```python
from build123d import *

# Parameters (mm, degrees)
BOSS_EXTRUDE1_DEPTH = 2
CUT_EXTRUDE1_REACH  = 43.449
SKETCH2_R           = 1
SKETCH3_W           = 42.8
SKETCH3_H           = 53.28
CUT_EXTRUDE2_DEPTH  = 1
SKETCH4_W           = 1.5
SKETCH4_H           = 57.28
BOSS_EXTRUDE2_DEPTH = 3.5
SKETCH5_W           = 1
SKETCH5_H           = 3
CUT_EXTRUDE3_DEPTH  = 16.633
CHAMFER1_SIZE       = 1
CHAMFER2_SIZE       = 2.5
CHAMFER3_SIZE       = 1.5
CHAMFER4_SIZE       = 1.5


# Some blends are built 0.0001 mm under size
with BuildPart() as part:
    # Sketch1 → Boss-Extrude1 (new body)
    with BuildSketch(Plane.XY):
        with BuildLine():
            Line((-23.2, -26.99), (-23.2, 27.29))
            ThreePointArc((-23.2, 27.29), (-22.702081528, 28.492081528), (-21.5, 28.99))
            Line((-21.5, 28.99), (-7.3, 28.99))
            ThreePointArc((-7.3, 28.99), (-5.673654403, 29.663654403), (-5, 31.29))
            Line((-5, 31.29), (-5, 32.59))
            ThreePointArc((-5, 32.59), (-4.502081528, 33.792081528), (-3.3, 34.29))
            Line((-3.3, 34.29), (1.7, 34.29))
            ThreePointArc((1.7, 34.29), (2.902081528, 33.792081528), (3.4, 32.59))
            Line((3.4, 32.59), (3.4, 31.29))
            ThreePointArc((3.4, 31.29), (4.073654403, 29.663654403), (5.7, 28.99))
            Line((5.7, 28.99), (19.9, 28.99))
            ThreePointArc((19.9, 28.99), (21.102081528, 28.492081528), (21.6, 27.29))
            Line((21.6, 27.29), (21.6, -26.99))
            Line((21.6, -26.99), (-23.2, -26.99))
        make_face()
    extrude(amount=BOSS_EXTRUDE1_DEPTH)

    # Sketch2 → Cut-Extrude1 (cut, up to next)
    with BuildSketch(Plane(origin=(0, 0, 0), x_dir=(-1, 0, 0), z_dir=(0, 0, -1)), mode=Mode.PRIVATE) as cut_extrude1_sk1:
        with Locations((0.8, 30.84)):
            Circle(SKETCH2_R)
    cut_extrude1_tool1 = extrude(cut_extrude1_sk1.sketch, amount=-CUT_EXTRUDE1_REACH, mode=Mode.PRIVATE) & part.part
    add(cut_extrude1_tool1.solids().sort_by_distance((-0.8, 30.84, 0))[0], mode=Mode.SUBTRACT)

    # Sketch3 → Cut-Extrude2 (cut)
    with BuildSketch(Plane(origin=(0, 0, 0), x_dir=(-1, 0, 0), z_dir=(0, 0, -1))):
        with Locations((0.8, 0.65)):
            Rectangle(SKETCH3_W, SKETCH3_H)
    extrude(amount=-CUT_EXTRUDE2_DEPTH, mode=Mode.SUBTRACT)

    # Sketch4 → Boss-Extrude2 (add)
    with BuildSketch(Plane(origin=(0, 0, 1), x_dir=(-1, 0, 0), z_dir=(0, 0, -1))):
        with Locations((-6.7665, -1.35)):
            Rectangle(SKETCH4_W, SKETCH4_H)
        with Locations((8.3665, -1.35)):
            Rectangle(SKETCH4_W, SKETCH4_H)
    extrude(amount=BOSS_EXTRUDE2_DEPTH)

    # Sketch5 → Cut-Extrude3 (cut)
    with BuildSketch(Plane(origin=(7.5165, 0, 0), x_dir=(0, 0, -1), z_dir=(1, 0, 0))):
        with Locations((-0.5, -28.49)):
            Rectangle(SKETCH5_W, SKETCH5_H)
    extrude(amount=-CUT_EXTRUDE3_DEPTH, mode=Mode.SUBTRACT)

    # Chamfer1
    chamfer1_edges = [part.edges().sort_by_distance(p)[0] for p in [
        (6.7665, -29.99, -2.5),
        (-8.3665, -29.99, -2.5),
    ]]
    chamfer(chamfer1_edges, length=CHAMFER1_SIZE)

    # Chamfer2
    chamfer2_edges = [part.edges().sort_by_distance(p)[0] for p in [
        (6.7665, 27.29, -2.5),
        (-8.3665, 27.29, -2.5),
    ]]
    chamfer(chamfer2_edges, length=CHAMFER2_SIZE - 0.0001)  # a hair under: the kernel refuses the full size

    # Chamfer3
    # the kernel refuses this chamfer: 1.5 mm, written as the material it takes off along each edge
    with BuildSketch(Plane(origin=(-7.157524482, 34.29, 0), x_dir=(0, -0.9996219169112968, -0.02749587661058636), z_dir=(1, 0, 0))) as chamfer3_piece_1:
        Polygon((CHAMFER3_SIZE * 0.999621916911, -CHAMFER3_SIZE * 0.0274958766106), (-CHAMFER3_SIZE * 0.0274958766106, -CHAMFER3_SIZE * 0.999621916911), (0, 0), align=None)
    extrude(amount=12.715048964, mode=Mode.SUBTRACT)

    # Chamfer4
    chamfer4_edges = [part.edges().sort_by_distance(p)[0] for p in [
        (0.2, 30.84, 2),
    ]]
    chamfer(chamfer4_edges, length=CHAMFER4_SIZE)


solid = part.part
```
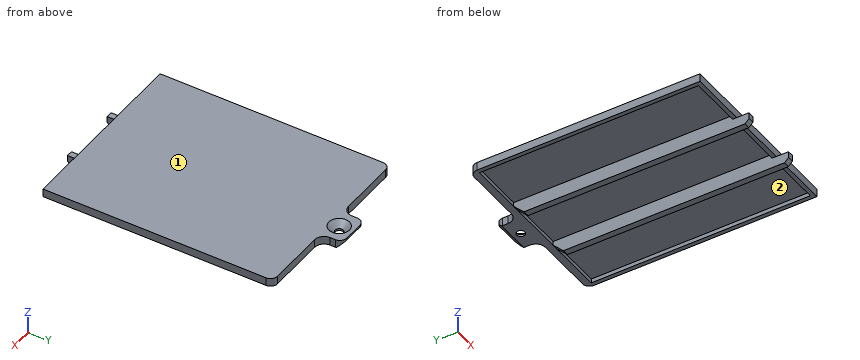
The listing builds one solid part. Answer for the finished solid, in the listing's coordinates (mm). Face numbers are marked on the shaded views. Round coordinates to 2 decimals unless told otherwise and drop trailing zeros. Loops run counter-clockwise (first coordinate to the right, second up) from the corner with the lowest first, then second, coordinate; pieces in that order, holes last. Notation, with made-up numbers: (61, -28) - (75, -28) arc R8 cw to (75, -24) - close; hole circle Ø8 at (83.5, 31). An arc over 180 degrees is marked (long way). Return JSON: item names as keys, results as strings. Group by question number.
1. The part is cut by section C-C on x = -14.5. Determine the outline of the cut face in (y, z), then the cut area to 3 significant figures.
2. The part is cut by section A-A on x = -0.8. Determine the outline of the cut face in (y, z).
3. Consider probe 1 along X at (y, z) = (5.5, 0.45); probe 2 along Y at (x, z) = (-0.8, 0.2); probe 3 along X at (y, z) = (21.5, -0.75). Determine where each line is inside the solid, lowest interval first.
4. The mould has two halves that part along Y. Classify the marked faces 1 and 2: pulls with the +Y half, pulls with the -Y half, needs draft (parallel to the pull), parting line crosses it, or undercut.
5. Each of these flat-tipped pins is pushed along its axis until it touches: P1, Ø0.6, axis at x = -2.5, z = 1.5, coming from the -Y side; P2, Ø1, axis at x = 16.5, z = -2, coming from the +Y side; P3, Ø4, axis at x = 17, y = -12, coming from the -Z side; P4, Ø0.5, axis at x = -2, y = -26.5, coming from the -Z side. Where does it stop, or does it pass through?
6. The part is cut by section D-D on y = 25.5. Determine the outline of the cut face in (x, z).
7. The part is cut by section B-B on y = 8.5. Determine the outline of the cut face in (x, z).
Resolved:
{
 "1": {"outline": "(-26.99, 0) - (-25.99, 0) - (-25.99, 1) - (27.29, 1) - (27.29, 0) - (28.99, 0) - (28.99, 2) - (-26.99, 2) - close", "area": "58.7 mm²"},
 "2": {"outline": "(-26.99, 0) - (-25.99, 0) - (-25.99, 1) - (27.29, 1) - (27.29, 0) - (29.84, 0) - (29.84, 0.5) - (28.34, 2) - (-26.99, 2) - close; (31.84, 0) - (32.79, 0) - (34.29, 1.5) - (34.29, 2) - (33.34, 2) - (31.84, 0.5) - close"},
 "3": {"probe 1": "x = -23.2 to -22.2, -9.12 to -7.62, 6.02 to 7.52, 20.6 to 21.6", "probe 2": "y = -26.99 to -25.99, 27.29 to 29.84, 31.84 to 32.99", "probe 3": "x = -9.12 to -7.62, 6.02 to 7.52"},
 "4": {"face 1": "needs draft", "face 2": "undercut"},
 "5": {"P1": "stops at y = -26.99", "P2": "passes through", "P3": "stops at z = 1", "P4": "stops at z = 0"},
 "6": {"outline": "(-23.2, 0) - (-22.2, 0) - (-22.2, 1) - (-9.12, 1) - (-9.12, -1.79) - (-7.62, -1.79) - (-7.62, 1) - (6.02, 1) - (6.02, -1.79) - (7.52, -1.79) - (7.52, 1) - (20.6, 1) - (20.6, 0) - (21.6, 0) - (21.6, 2) - (-23.2, 2) - close"},
 "7": {"outline": "(-23.2, 0) - (-22.2, 0) - (-22.2, 1) - (-9.12, 1) - (-9.12, -2.5) - (-7.62, -2.5) - (-7.62, 1) - (6.02, 1) - (6.02, -2.5) - (7.52, -2.5) - (7.52, 1) - (20.6, 1) - (20.6, 0) - (21.6, 0) - (21.6, 2) - (-23.2, 2) - close"}
}
